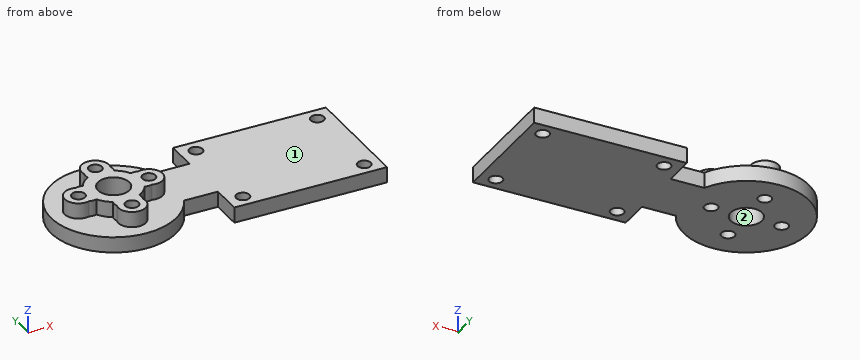
from build123d import *

# Parameters (mm, degrees)
METAL_HORN_FLANGE_PROFILE_R              = 16
METAL_HORN_FLANGE_DEPTH                  = 4
STRAIGHT_FOREARM_WEB_PROFILE_W           = 28
STRAIGHT_FOREARM_WEB_PROFILE_H           = 14
STRAIGHT_FOREARM_WEB_DEPTH               = 4
REPLACEABLE_TOOL_MOUNTING_DECK_PROFILE_W = 39
REPLACEABLE_TOOL_MOUNTING_DECK_PROFILE_H = 30
REPLACEABLE_TOOL_MOUNTING_DECK_DEPTH     = 4
DOWEL_SUPPORT_HUB_START                  = 4
DOWEL_SUPPORT_HUB_PROFILE_R              = 7
DOWEL_SUPPORT_HUB_PROFILE_R_2            = 4
DOWEL_SUPPORT_HUB_DEPTH                  = 4
WASHER_SEATS_CLEAR_DOWEL_SLEEVE_START    = 4
RAISED_WASHER_SEATS_PCD14_R              = 3.5
WASHER_SEATS_CLEAR_DOWEL_SLEEVE_DEPTH    = 4
ELBOW_SLEEVE_BORE_START                  = -50
ELBOW_SLEEVE_BORE_PROFILE_R              = 4
ELBOW_SLEEVE_BORE_DEPTH                  = 115.52906322
MODULAR_TOOL_FOUR_M3_PATTERN_START       = -50
MODULAR_TOOL_FOUR_M3_PATTERN_PROFILE_R   = 1.7
MODULAR_TOOL_FOUR_M3_PATTERN_DEPTH       = 115.52906322
PRINTED_HUB_M3_WASHER_SEATS_PCD18_START  = 4
PRINTED_HUB_WASHER_SEATS_PCD18_PROFILE_R = 3.5
PRINTED_HUB_M3_WASHER_SEATS_PCD18_DEPTH  = 4
PRINTED_HUB_M3_CLEARANCE_PCD18_START     = -50
PRINTED_HUB_M3_CLEARANCE_PCD18_PROFILE_R = 1.7
PRINTED_HUB_M3_CLEARANCE_PCD18_DEPTH     = 115.52906322


with BuildPart() as part:
    # Metal_horn_flange_profile → Metal_horn_flange (new body)
    with BuildSketch(Plane.XY):
        Circle(METAL_HORN_FLANGE_PROFILE_R)
    extrude(amount=METAL_HORN_FLANGE_DEPTH)

    # Straight_forearm_web_profile → Straight_forearm_web (add)
    with BuildSketch(Plane.XY):
        with Locations((14, 0)):
            Rectangle(STRAIGHT_FOREARM_WEB_PROFILE_W, STRAIGHT_FOREARM_WEB_PROFILE_H)
    extrude(amount=STRAIGHT_FOREARM_WEB_DEPTH)

    # Replaceable_tool_mounting_deck_profile → Replaceable_tool_mounting_deck (add)
    with BuildSketch(Plane.XY):
        with Locations((42.5, 0)):
            Rectangle(REPLACEABLE_TOOL_MOUNTING_DECK_PROFILE_W, REPLACEABLE_TOOL_MOUNTING_DECK_PROFILE_H)
    extrude(amount=REPLACEABLE_TOOL_MOUNTING_DECK_DEPTH)

    # Dowel_support_hub_profile → Dowel_support_hub (add)
    with BuildSketch(Plane.XY.offset(DOWEL_SUPPORT_HUB_START)):
        Circle(DOWEL_SUPPORT_HUB_PROFILE_R)
        Circle(DOWEL_SUPPORT_HUB_PROFILE_R_2, mode=Mode.SUBTRACT)
    extrude(amount=DOWEL_SUPPORT_HUB_DEPTH)

    # Raised_washer_seats_PCD14 → Washer_seats_clear_dowel_sleeve (add)
    with BuildSketch(Plane.XY.offset(WASHER_SEATS_CLEAR_DOWEL_SLEEVE_START)):
        with Locations((7, 0)):
            Circle(RAISED_WASHER_SEATS_PCD14_R)
        with Locations((-7, 0)):
            Circle(RAISED_WASHER_SEATS_PCD14_R)
        with Locations((0, 7)):
            Circle(RAISED_WASHER_SEATS_PCD14_R)
        with Locations((0, -7)):
            Circle(RAISED_WASHER_SEATS_PCD14_R)
    extrude(amount=WASHER_SEATS_CLEAR_DOWEL_SLEEVE_DEPTH)

    # Elbow_sleeve_bore_profile → Elbow_sleeve_bore (cut, through all)
    with BuildSketch(Plane.XY.offset(ELBOW_SLEEVE_BORE_START)):
        Circle(ELBOW_SLEEVE_BORE_PROFILE_R)
    extrude(amount=ELBOW_SLEEVE_BORE_DEPTH, mode=Mode.SUBTRACT)

    # Modular_tool_four_M3_pattern_profile → Modular_tool_four_M3_pattern (cut, through all)
    with BuildSketch(Plane.XY.offset(MODULAR_TOOL_FOUR_M3_PATTERN_START)):
        with Locations(Location((27, -11.5, 0), (0, 0, 180))):
            Circle(MODULAR_TOOL_FOUR_M3_PATTERN_PROFILE_R)
        with Locations(Location((27, 11.5, 0), (0, 0, 180))):
            Circle(MODULAR_TOOL_FOUR_M3_PATTERN_PROFILE_R)
        with Locations(Location((58, -11.5, 0), (0, 0, 180))):
            Circle(MODULAR_TOOL_FOUR_M3_PATTERN_PROFILE_R)
        with Locations(Location((58, 11.5, 0), (0, 0, 180))):
            Circle(MODULAR_TOOL_FOUR_M3_PATTERN_PROFILE_R)
    extrude(amount=MODULAR_TOOL_FOUR_M3_PATTERN_DEPTH, mode=Mode.SUBTRACT)

    # Printed_hub_washer_seats_PCD18_profile → Printed_hub_M3_washer_seats_PCD18 (add)
    with BuildSketch(Plane.XY.offset(PRINTED_HUB_M3_WASHER_SEATS_PCD18_START)):
        with Locations((9, 0)):
            Circle(PRINTED_HUB_WASHER_SEATS_PCD18_PROFILE_R)
        with Locations((0, 9)):
            Circle(PRINTED_HUB_WASHER_SEATS_PCD18_PROFILE_R)
        with Locations((-9, 0)):
            Circle(PRINTED_HUB_WASHER_SEATS_PCD18_PROFILE_R)
        with Locations((0, -9)):
            Circle(PRINTED_HUB_WASHER_SEATS_PCD18_PROFILE_R)
    extrude(amount=PRINTED_HUB_M3_WASHER_SEATS_PCD18_DEPTH)

    # Printed_hub_M3_clearance_PCD18_profile → Printed_hub_M3_clearance_PCD18 (cut, through all)
    with BuildSketch(Plane.XY.offset(PRINTED_HUB_M3_CLEARANCE_PCD18_START)):
        with Locations(Location((9, 0, 0), (0, 0, 180))):
            Circle(PRINTED_HUB_M3_CLEARANCE_PCD18_PROFILE_R)
        with Locations(Location((0, 9, 0), (0, 0, 180))):
            Circle(PRINTED_HUB_M3_CLEARANCE_PCD18_PROFILE_R)
        with Locations(Location((-9, 0, 0), (0, 0, 180))):
            Circle(PRINTED_HUB_M3_CLEARANCE_PCD18_PROFILE_R)
        with Locations(Location((0, -9, 0), (0, 0, 180))):
            Circle(PRINTED_HUB_M3_CLEARANCE_PCD18_PROFILE_R)
    extrude(amount=PRINTED_HUB_M3_CLEARANCE_PCD18_DEPTH, mode=Mode.SUBTRACT)


solid = part.part
CAD build for the part. Positions are in the model's coordinates, mm. Face numbers are marked on the shaded views. Round coordinates to 2 decimals unless told otherwise and drop trailing zeros. Order: outer loops, then holes, each group sorted by start corner. A loop starts at its lowest first (then second) coordinate and runs counter-clockwise, first axis right, second up. Notation, with made-up numbers: M 74,46 L 88,46 A22 ccw 88,78 Z; hole C -39.75,48.25 d7. An arc over 180 degrees is marked long. Use one line per item in the form item = value.
Q1. Saw through at C-C on z = 2.5. State how many separate pieces and enclosed holes the cut face has, then the cut area to 3 significant figures.
Recorded:
separate_pieces = 1
enclosed_holes = 9
area = 1,960 mm^2
Q2. Saw through at A-A on y = 0. Give the cut face in (x, z).
Recorded:
outline = M -16,0 L -10.7,0 L -10.7,8 L -12.5,8 L -12.5,4 L -16,4 Z; M -7.3,0 L -4,0 L -4,8 L -7.3,8 Z; M 4,0 L 7.3,0 L 7.3,8 L 4,8 Z; M 10.7,0 L 62,0 L 62,4 L 12.5,4 L 12.5,8 L 10.7,8 Z
Q3. Saw through at B-B on x = 58. Give the cut face in (y, z).
Recorded:
outline = M -15,0 L -13.2,0 L -13.2,4 L -15,4 Z; M -9.8,0 L 9.8,0 L 9.8,4 L -9.8,4 Z; M 13.2,0 L 15,0 L 15,4 L 13.2,4 Z
Q4. Saw through at D-D on y = 9. Give the cut face in (x, z).
Recorded:
outline = M -13.23,0 L -1.7,0 L -1.7,8 L -3.5,8 L -3.5,4 L -13.23,4 Z; M 1.7,0 L 13.23,0 L 13.23,4 L 3.5,4 L 3.5,8 L 1.7,8 Z; M 23,0 L 62,0 L 62,4 L 23,4 Z
Q5. Probe L1, parallel to Y at x = 0, z = 6.25; L2, parallel to Y at x = 27, z = 2.9; L3, parallel to X at y = 13, z = 1.25. List the from-to ranges inside material, lowest first.
Recorded:
L1 = -12.5 to -10.7, -7.3 to -4, 4 to 7.3, 10.7 to 12.5
L2 = -15 to -13.2, -9.8 to 9.8, 13.2 to 15
L3 = -9.33 to 9.33, 23 to 26.2, 27.8 to 57.2, 58.8 to 62
Q6. Two-plate mould, pull along X, no slides. Class the marked faces 1 and 2: +X half, -X half, draft (parallel to the pull), parting line (faces both ways), or undercut.
Recorded:
face_1 = draft
face_2 = undercut
Q7. Flat gauge pins, fed straight in: P1, Ø1.2, axis at y = 12, z = 1.5, coming from the -X side; P2, Ø2, axis at x = 44, z = 3, coming from the -Y side; P3, Ø4, axis at x = 13.5, y = -2.5, coming from the -Z side; P4, Ø2.5, axis at x = 0, y = 9, coming from the -Z side. Where does each tip first touch, or does it go through?
Recorded:
P1 = -11.23
P2 = -15
P3 = 0
P4 = through
